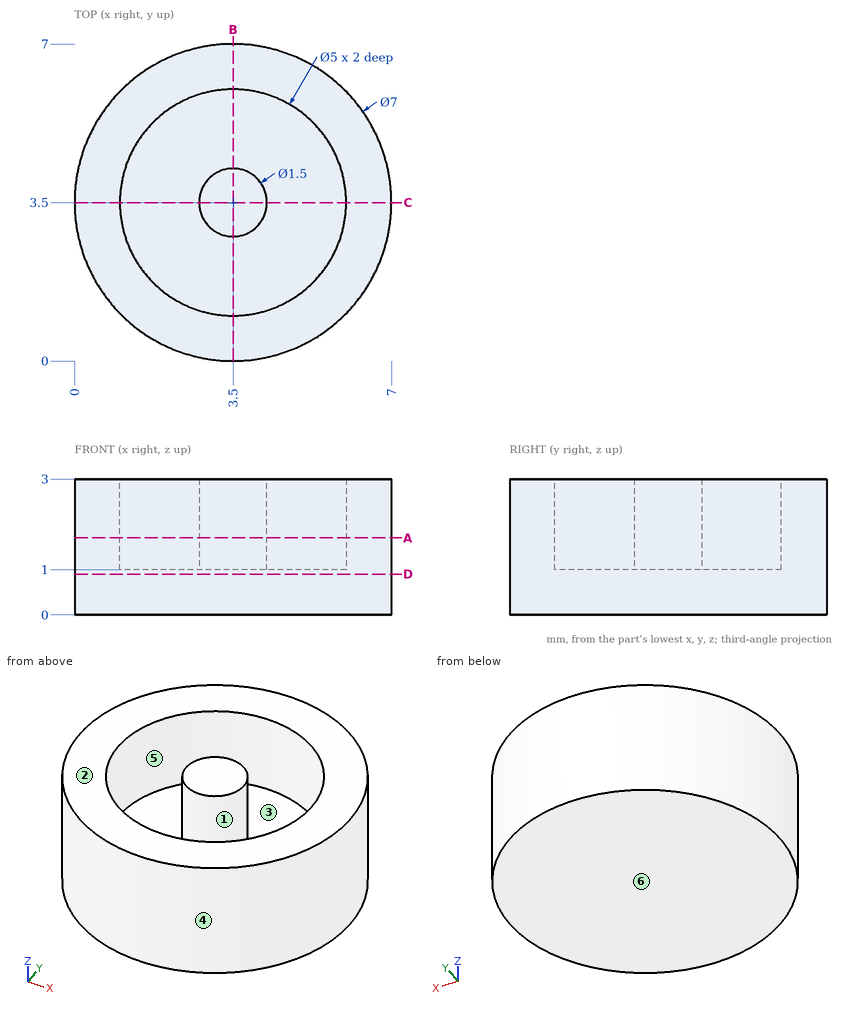
Drawing for the job (mm, zero at the part's lowest x, y, z). A direction names the side the tool comes from. Round coordinates to 2 decimals unless told otherwise and drop trailing zeros. Loops run counter-clockwise (first coordinate to the right, second up) from the corner with the lowest first, then second, coordinate; pieces in that order, holes last.
1. Mould opens along X. For the marked faces 3, 4, 5 and 6 say: +X half, -X half, draft (parallel to the pull), parting line (faces both ways), or undercut.
Check values:
face 3: undercut
face 4: parting line
face 5: undercut
face 6: draft
2. Band-saw the part on D-D, the plane z = 0.9. List the corners of the cut face in (x, y).
Check values:
outline: circle Ø7 at (3.5, 3.5)
3. Wall check: probe 1 along Y at (x, z) = (3.5, 2.15); probe 2 along Z at (x, y) = (1.5, 2.25); probe 3 along X at (y, z) = (5.5, 2.2). Give the ranges that are in metal, low to high.
Check values:
probe 1: y = 0 to 1, 2.75 to 4.25, 6 to 7
probe 2: z = 0 to 1
probe 3: x = 0.63 to 2, 5 to 6.37
4. Band-saw the part on B-B, the plane x = 3.5. List the corners of the cut face in (y, z).
Check values:
outline: (0, 0) - (7, 0) - (7, 3) - (6, 3) - (6, 1) - (4.25, 1) - (4.25, 3) - (2.75, 3) - (2.75, 1) - (1, 1) - (1, 3) - (0, 3) - close
5. Tool access for the marked faces 1 and 2: list every direction of +Z, -Z, +X, -X, +Y, -Y with a clear straight run to the whole face (end or side of a thin tool).
Check values:
face 1: +Z
face 2: +Z, +X, -X, +Y, -Y
6. Band-saw the part on A-A, the plane z = 1.7. List the corners of the cut face in (x, y).
Check values:
outline: circle Ø7 at (3.5, 3.5); circle Ø1.5 at (3.5, 3.5); hole circle Ø5 at (3.5, 3.5)
